Part model, mm, in its own coordinate system. Face numbers are marked on the shaded views. A direction names the side the tool comes from. Coordinates: 2 decimals unless noted, no trailing zeros. Loops run counter-clockwise (first coordinate to the right, second up) from the corner with the lowest first, then second, coordinate; pieces in that order, holes last. Notation, with made-up numbers: (-40, -20.5) - (-22, -20.5) arc R16 ccw to (-22, 6.5) - close; hole circle Ø4 at (67.5, 3.25). An arc over 180 degrees is marked (long way). Use a Markdown table: item, result. Add a question column.
1) Band-saw the part on C-C (z = 0). Give the number of separate pieces and of enclosed holes in the cut face, plus the area to 3 significant figures.
2) Probe probe 1 along Z at (x, y) = (-40, 17); probe 2 along Y at (x, z) = (-32.5, 9); probe 3 along X at (y, z) = (-17, 7). List the from-to ranges inside material, lowest first. Write a range as [from, to].
3) Band-saw the part on A-A (x = 250). Give the cut face in (y, z), plus the area to 3 significant figures.
4) Pull direction X, two halves, no side cores. Call the marked faces 4, 5 and 6: +X half, -X half, draft (parallel to the pull), parting line (faces both ways), or undercut.
5) Drop flat-ended pins along their axis: P1, Ø8, axis at x = 100.5, y = -16.5, coming from the -Z side; P2, Ø10, axis at x = 232, z = 7, coming from the -Y side; P3, Ø13, axis at x = 15, z = -43, coming from the +Y side. Give the stop position or say it passes through.
6) Band-saw the part on D-D (y = -27). Give the cut face in (x, z).
7) Tool access for the marked faces 1, 2 and 3: list every direction of +Z, -Z, +X, -X, +Y, -Y with a clear straight run to the whole face (end or side of a thin tool).
8) Band-saw the part on B-B (y = 6). Give the cut face in (x, z), plus the area to 3 significant figures.
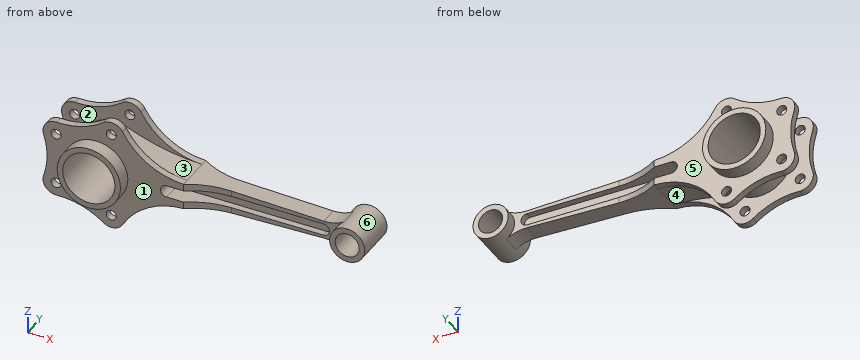
from build123d import *

# Parameters (mm, degrees)
SKETCH1_R               = 31.5
SKETCH1_R_2             = 26
BOSS_EXTRUDE1_DEPTH     = 35
SKETCH1_3_R             = 31.5
SKETCH1_3_R_2           = 26
BOSS_EXTRUDE2_DEPTH     = 21
SKETCH2_R               = 5
BOSS_EXTRUDE7_DEPTH     = 21
CUT_EXTRUDE3_DEPTH      = 250.349008072
CUT_EXTRUDE3_DEPTH_BACK = 250.349008072
SKETCH2_6_R             = 17.5
SKETCH2_6_R_2           = 12
BOSS_EXTRUDE8_DEPTH     = 21
CUT_EXTRUDE4_START      = 2.5
CUT_EXTRUDE4_DEPTH      = 18.5
CUT_EXTRUDE5_DEPTH      = 14
CUT_EXTRUDE7_DEPTH      = 276.530851267
CUT_EXTRUDE7_DEPTH_BACK = 276.530851267
SKETCH1_5_R             = 26


# Read off the part's stored shape, not the designer's step: Cut-Extrude4
with BuildPart() as part:
    # Sketch1 → Boss-Extrude1 (new, symmetric)
    with BuildSketch(Plane(origin=(0, 0, 0), x_dir=(1, 0, 0), z_dir=(0, 1, 0))):
        with Locations(Location((0, 0, 0), (0, 0, 270))):
            Circle(SKETCH1_R)
        with Locations(Location((0, 0, 0), (0, 0, 270))):
            Circle(SKETCH1_R_2, mode=Mode.SUBTRACT)
    extrude(amount=BOSS_EXTRUDE1_DEPTH, both=True)

    # Sketch1<3> → Boss-Extrude2 (add, symmetric)
    with BuildSketch(Plane(origin=(0, 0, 0), x_dir=(1, 0, 0), z_dir=(0, 1, 0))):
        with Locations(Location((0, 0, 0), (0, 0, 270))):
            Circle(SKETCH1_3_R)
        with Locations(Location((0, 0, 0), (0, 0, 270))):
            Circle(SKETCH1_3_R_2, mode=Mode.SUBTRACT)
    extrude(amount=BOSS_EXTRUDE2_DEPTH, both=True)

    # Sketch2 → Boss-Extrude7 (add, symmetric)
    with BuildSketch(Plane(origin=(0, 0, 0), x_dir=(1, 0, 0), z_dir=(0, 1, 0))):
        with BuildLine():
            Line((220.285908843, 9), (87, 13))
            ThreePointArc((87, 13), (51.867643982, 23.236099658), (26.304344234, 49.419641847))
            ThreePointArc((26.304344234, 49.419641847), (17.640533854, 55.729005498), (7.181946677, 53.386435492))
            ThreePointArc((7.181946677, 53.386435492), (-14.855989459, 42.122318837), (-39.406288617, 38.986435492))
            ThreePointArc((-39.406288617, 38.986435492), (-50.326951915, 33.896458963), (-52.376901133, 22.023529412))
            ThreePointArc((-52.376901133, 22.023529412), (-48.925892025, 0), (-52.376901133, -22.023529412))
            ThreePointArc((-52.376901133, -22.023529412), (-50.326951915, -33.896458963), (-39.406288617, -38.986435492))
            ThreePointArc((-39.406288617, -38.986435492), (-14.855989459, -42.122318837), (7.181946677, -53.386435492))
            ThreePointArc((7.181946677, -53.386435492), (17.640533854, -55.729005498), (26.304344234, -49.419641847))
            ThreePointArc((26.304344234, -49.419641847), (51.867643982, -23.236099658), (87, -13))
            Line((87, -13), (220.285908843, -9))
            ThreePointArc((220.285908843, -9), (230.798886909, -10.287807913), (240.445269919, -14.661416476))
            ThreePointArc((240.445269919, -14.661416476), (232.5, 0), (240.445269919, 14.661416476))
            ThreePointArc((240.445269919, 14.661416476), (230.798886909, 10.287807913), (220.285908843, 9))
        make_face()
        with Locations(Location((15, 43, 0), (0, 0, 90))):
            Circle(SKETCH2_R, mode=Mode.SUBTRACT)
        with Locations(Location((15, -43, 0), (0, 0, 90))):
            Circle(SKETCH2_R, mode=Mode.SUBTRACT)
        with Locations(Location((-40, -26, 0), (0, 0, 90))):
            Circle(SKETCH2_R, mode=Mode.SUBTRACT)
        with Locations(Location((-40, 26, 0), (0, 0, 90))):
            Circle(SKETCH2_R, mode=Mode.SUBTRACT)
    extrude(amount=BOSS_EXTRUDE7_DEPTH, both=True)

    # Sketch6 → Cut-Extrude3 (cut, two sides: drawn at the far end of the back side and taken through both)
    with BuildSketch(Plane.XY.offset(-CUT_EXTRUDE3_DEPTH_BACK)):
        with BuildLine():
            Line((240.445269919, 21), (220.285908843, 21))
            Line((220.285908843, 21), (87, 21))
            ThreePointArc((87, 21), (106.935911729, 12.060024019), (128.569219382, 9))
            Line((128.569219382, 9), (240.445269919, 9))
            Line((240.445269919, 9), (240.445269919, 21))
        make_face()
        with BuildLine():
            Line((240.445269919, -9), (128.569219382, -9))
            ThreePointArc((128.569219382, -9), (106.935911729, -12.060024019), (87, -21))
            Line((87, -21), (240.445269919, -21))
            Line((240.445269919, -21), (240.445269919, -9))
        make_face()
    extrude(amount=CUT_EXTRUDE3_DEPTH + CUT_EXTRUDE3_DEPTH_BACK, mode=Mode.SUBTRACT)

    # Sketch2<6> → Boss-Extrude8 (add, symmetric)
    with BuildSketch(Plane(origin=(0, 0, 0), x_dir=(1, 0, 0), z_dir=(0, 1, 0))):
        with Locations(Location((250, 0, 0), (0, 0, 270))):
            Circle(SKETCH2_6_R)
        with Locations(Location((250, 0, 0), (0, 0, 90))):
            Circle(SKETCH2_6_R_2, mode=Mode.SUBTRACT)
    extrude(amount=BOSS_EXTRUDE8_DEPTH, both=True)

    # Cut-Extrude4 outline → Cut-Extrude4 (cut)
    with BuildSketch(Plane(origin=(0, 0, 0), x_dir=(1, 0, 0), z_dir=(0, 1, 0)).offset(CUT_EXTRUDE4_START)):
        with BuildLine():
            ThreePointArc((220, -6), (226, 0), (220, 6))
            Line((220, 6), (70, 6))
            ThreePointArc((70, 6), (64, 0), (70, -6))
            Line((70, -6), (220, -6))
        make_face()
    cut_extrude4 = extrude(amount=CUT_EXTRUDE4_DEPTH, mode=Mode.SUBTRACT)

    # Mirror3: Cut-Extrude4 across plane
    add(cut_extrude4.mirror(Plane.ZX), mode=Mode.SUBTRACT)

    # Sketch9 → Cut-Extrude5 (cut, symmetric)
    with BuildSketch(Plane(origin=(0, 0, 0), x_dir=(1, 0, 0), z_dir=(0, 1, 0))):
        with BuildLine():
            ThreePointArc((87, -13), (48.833727891, -17.562334102), (12.155663261, -29.060107548))
            ThreePointArc((12.155663261, -29.060107548), (-31.5, 0), (12.155663261, 29.060107548))
            ThreePointArc((12.155663261, 29.060107548), (48.833727891, 17.562334102), (87, 13))
            ThreePointArc((87, 13), (51.867643982, 23.236099658), (26.304344234, 49.419641847))
            ThreePointArc((26.304344234, 49.419641847), (17.640533854, 55.729005498), (7.181946677, 53.386435492))
            ThreePointArc((7.181946677, 53.386435492), (-14.855989459, 42.122318837), (-39.406288617, 38.986435492))
            ThreePointArc((-39.406288617, 38.986435492), (-50.326951915, 33.896458963), (-52.376901133, 22.023529412))
            ThreePointArc((-52.376901133, 22.023529412), (-48.925892025, 0), (-52.376901133, -22.023529412))
            ThreePointArc((-52.376901133, -22.023529412), (-50.326951915, -33.896458963), (-39.406288617, -38.986435492))
            ThreePointArc((-39.406288617, -38.986435492), (-14.855989459, -42.122318837), (7.181946677, -53.386435492))
            ThreePointArc((7.181946677, -53.386435492), (17.640533854, -55.729005498), (26.304344234, -49.419641847))
            ThreePointArc((26.304344234, -49.419641847), (51.867643982, -23.236099658), (87, -13))
        make_face()
    extrude(amount=CUT_EXTRUDE5_DEPTH, both=True, mode=Mode.SUBTRACT)

    # Sketch1<5> → Cut-Extrude7 (cut, two sides: drawn at the far end of the back side and taken through both)
    with BuildSketch(Plane(origin=(0, 0, 0), x_dir=(1, 0, 0), z_dir=(0, 1, 0)).offset(-CUT_EXTRUDE7_DEPTH_BACK)):
        with Locations(Location((0, 0, 0), (0, 0, 270))):
            Circle(SKETCH1_5_R)
    extrude(amount=CUT_EXTRUDE7_DEPTH + CUT_EXTRUDE7_DEPTH_BACK, mode=Mode.SUBTRACT)


solid = part.part
Answer block:
| question | item | result |
|---|---|---|
| 1 | separate pieces | 3 |
| 1 | enclosed holes | 0 |
| 1 | area | 3,770 mm2 |
| 2 | probe 1 | [-39, -31], [-21, 21], [31, 39] |
| 2 | probe 2 | [-21, -14], [14, 21] |
| 2 | probe 3 | [-49.27, -25.04], [25.04, 94.16], [233.96, 240.25], [259.75, 266.04] |
| 3 | outline | (-21, -17.5) - (21, -17.5) - (21, -12) - (-21, -12) - close; (-21, 12) - (21, 12) - (21, 17.5) - (-21, 17.5) - close |
| 3 | area | 462 mm2 |
| 4 | face 4 | undercut |
| 4 | face 5 | draft |
| 4 | face 6 | undercut |
| 5 | P1 | z = -12.71 |
| 5 | P2 | y = -21 |
| 5 | P3 | y = 21 |
| 6 | outline | circle Ø63 at (0, 0); hole circle Ø52 at (0, 0) |
| 7 | face 1 | -Y |
| 7 | face 2 | none |
| 7 | face 3 | +Z |
| 8 | outline | (12.16, -29.06) arc R208.29 cw to (87, -13) - (220.29, -9) arc R35 cw to (240.45, -14.66) arc R17.5 ccw (long way) to (240.45, 14.66) arc R35 cw to (220.29, 9) - (87, 13) arc R208.29 cw to (12.16, 29.06) arc R31.5 ccw (long way) to start; hole circle Ø52 at (0, 0); hole (70, -6) - (220, -6) arc R6 ccw to (220, 6) - (70, 6) arc R6 ccw to start; hole circle Ø24 at (250, 0) |
| 8 | area | 4,760 mm2 |
